```python
from build123d import *

# Parameters (mm, degrees)
F0_W        = 100
F0_H        = 20
F1_DEPTH    = 2
F2_R        = 15
F4_DEPTH    = 25
F5_T1_DEPTH = 25
F5_T3_DEPTH = 50.9807621135
F5_T5_DEPTH = 50.9793707428
F5_T7_DEPTH = 55
F6_R        = 5
F8_D        = 7


# Not quite as in the source:
# - a fillet or chamfer that OpenCascade refuses, or shapes differently, is made with other operations: its cross-section is extruded or revolved along the edge and cut away or added


with BuildPart() as f1:
    # F0 (on Top) → F1 (new body)
    with BuildSketch(Plane.XY):
        with Locations((46.6617465019, -62.7806016803)):
            Rectangle(F0_W, F0_H)
    extrude(amount=F1_DEPTH)

    # F2
    f2_edges = [f1.edges().sort_by_distance(p)[0] for p in [
        (-3.338253, -52.780602, 1),
    ]]
    fillet(f2_edges, radius=F2_R)

    # F3 (on face) → F4 (join)
    with BuildSketch(Plane.XY.offset(2)):
        Polygon((-10.4593388438, -72.7806016803), (9.5406611562, -72.7806016803), (9.5406611562, -69.7806016803), (-10.4593388438, -69.7806016803), (-13.4593388438, -69.7806016803), (-13.4593388438, -72.7806016803), (-50.4598207772, -72.7806016803), (-50.4598207772, -69.7806016803), (-53.4593388438, -69.7806016803), (-53.4593388438, -72.7806016803), (-53.4593388438, -75.7806016803), (-50.4598207772, -75.7806016803), (-13.4593388438, -75.7806016803), (-10.4593388438, -75.7806016803), align=None)
    extrude(amount=F4_DEPTH)

    # F5: fillet of radius 6 on 5 edges, made by hand

    # F5_s2 → F5_t1 (join)
    with BuildSketch(Plane.XY.offset(2)):
        with BuildLine():
            ThreePointArc((-13.4593388438, -69.7806016803), (-15.6554912665, -71.976754103), (-18.6554912665, -72.7806016803))
            Line((-18.6554912665, -72.7806016803), (-13.4593388438, -72.7806016803))
            Line((-13.4593388438, -72.7806016803), (-13.4593388438, -69.7806016803))
        make_face()
        with BuildLine():
            ThreePointArc((-50.4598207772, -69.7806016803), (-48.2636683545, -71.976754103), (-45.2636683545, -72.7806016803))
            Line((-45.2636683545, -72.7806016803), (-50.4598207772, -72.7806016803))
            Line((-50.4598207772, -72.7806016803), (-50.4598207772, -69.7806016803))
        make_face()
    extrude(amount=F5_T1_DEPTH)

    # F5_s4 → F5_t3 (cut)
    with BuildSketch(Plane.XY.offset(-10.9903810568)):
        with BuildLine():
            ThreePointArc((-10.4593388438, -72.7806016803), (-12.6554912665, -74.976754103), (-15.6554912665, -75.7806016803))
            Line((-15.6554912665, -75.7806016803), (-10.4593388438, -75.7806016803))
            Line((-10.4593388438, -75.7806016803), (-10.4593388438, -72.7806016803))
        make_face()
    extrude(amount=F5_T3_DEPTH, mode=Mode.SUBTRACT)

    # F5_s6 → F5_t5 (cut)
    with BuildSketch(Plane.XY.offset(-10.9896853714)):
        with BuildLine():
            ThreePointArc((-53.4593388438, -74.9764758288), (-52.6556303868, -71.9767168052), (-50.4598207772, -69.7806016803))
            Line((-50.4598207772, -69.7806016803), (-53.4593388438, -69.7806016803))
            Line((-53.4593388438, -69.7806016803), (-53.4593388438, -74.9764758288))
        make_face()
    extrude(amount=F5_T5_DEPTH, mode=Mode.SUBTRACT)

    # F5_s8 → F5_t7 (cut)
    with BuildSketch(Plane.XY.offset(-13)):
        with BuildLine():
            ThreePointArc((-47.4593388438, -75.7806016803), (-51.7019795309, -74.0232423674), (-53.4593388438, -69.7806016803))
            Line((-53.4593388438, -69.7806016803), (-53.4593388438, -75.7806016803))
            Line((-53.4593388438, -75.7806016803), (-47.4593388438, -75.7806016803))
        make_face()
    extrude(amount=F5_T7_DEPTH, mode=Mode.SUBTRACT)

    # F6
    f6_edges = [f1.edges().sort_by_distance(p)[0] for p in [
        (9.540661, -71.280602, 27),
    ]]
    fillet(f6_edges, radius=F6_R)

    # F8 (through all)
    with Locations(Plane.XZ.offset(72.7806016803)):
        with Locations((-0.4593388438, 14.5)):
            Hole(F8_D / 2)


solid = f1.part
```
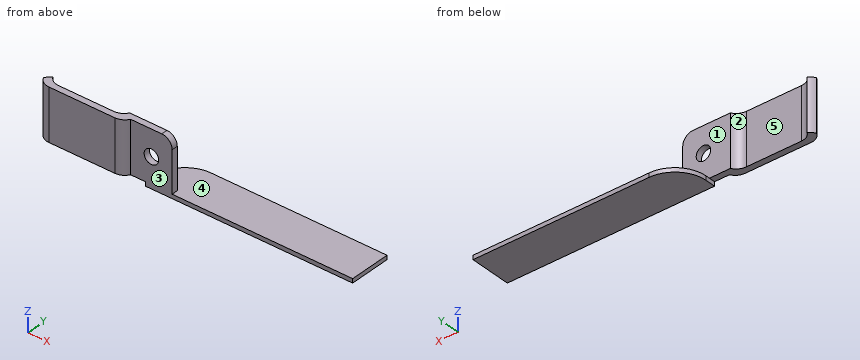
Geometry: final body of the model. Coordinates: model frame, mm. Face numbers are marked on the shaded views. A direction names the side the tool comes from. Coordinates: 2 decimals unless noted, no trailing zeros. Write each loop counter-clockwise with the first axis right and the second up, starting at its lowest first coordinate (ties: lowest second). Pieces come first, ordered by that corner, then holes. Notation, with made-up numbers: M 30,49.5 L 45,49.5 A30 ccw 45,88.5 Z; hole C -2.75,-22.5 d8. An arc over 180 degrees is marked long. Use CSV: the item, a comma, the result in double quotes. Start each with the question number.
1. Cut plane B-B on z = 5. Return the cut outline in (x, y).
2. First-contact query: P1, Ø8, axis at y = -63.5, z = 3.5, coming from the -X side; P2, Ø10, axis at y = -66.5, z = 13.5, coming from the +X side; P3, Ø2, axis at x = 44.5, y = -55.5, coming from the +Z side. Flat tips, straight axial feed; report the tip coordinate or a pass-through.
3. Reachability of the marked faces 1, 2 and 3 from +Z, -Z, +X, -X, +Y, -Y: full face, straight path, thin tool, end or side. Return the list, or none.
4. Ray query, probe 1 along Y at (x, z) = (-25, 6); probe 2 along Z at (x, y) = (11, -60.25); probe 3 along Z at (x, y) = (-34, -75). Return the intervals inside material, ascending.
5. Cut plane D-D on y = -63.5. Return the cut outline in (x, z), plus the area to 3 significant figures.
6. Cut plane C-C on x = -23. Return the cut outline in (y, z).
7. Mould query, pull axis X, two halves, no side actions, for the marked faces 4 and 5. Classes: pulls with the +X half, pulls with the -X half, needs draft (parallel to the pull), parting line crosses it, or undercut.
8. Cut plane A-A on z = 14.5. Return the cut outline in (x, y), plus the area to 3 significant figures.
Entries:
1,outline,"M -52.87,-72.38 A6 ccw -47.46,-75.78 L -15.66,-75.78 A6 ccw -10.46,-72.78 L 9.54,-72.78 L 9.54,-69.78 L -13.46,-69.78 A6 cw -18.66,-72.78 L -45.26,-72.78 A6 cw -50.46,-69.78 A6 ccw Z"
2,P1,"x = -3.33"
2,P2,"x = 9.54"
2,P3,"z = 2"
3,face 1,"+Z, +X, -X, +Y"
3,face 2,"+Z, -Z, +Y"
3,face 3,"+Z, -Z, +X, -Y"
4,probe 1,"-75.78 to -72.78"
4,probe 2,"0 to 2"
4,probe 3,"2 to 27"
5,outline,"M -2.71,0 L 96.66,0 L 96.66,2 L -2.71,2 Z"
5,area,"199 mm²"
6,outline,"M -75.78,2 L -72.78,2 L -72.78,27 L -75.78,27 Z"
7,face 4,"needs draft"
7,face 5,"undercut"
8,outline,"M -52.87,-72.38 A6 ccw -47.46,-75.78 L -15.66,-75.78 A6 ccw -10.46,-72.78 L -3.96,-72.78 L -3.96,-69.78 L -13.46,-69.78 A6 cw -18.66,-72.78 L -45.26,-72.78 A6 cw -50.46,-69.78 A6 ccw Z; M 3.04,-72.78 L 9.54,-72.78 L 9.54,-69.78 L 3.04,-69.78 Z"
8,area,"179 mm²"
